```python
from build123d import *

# Parameters (mm, degrees)
SKETCH_R      = 4
EXTRUDE_DEPTH = 10


with BuildPart() as part:
    # Sketch → Extrude (new body)
    with BuildSketch(Plane.XY):
        with BuildLine():
            Line((18.316745, 55.716924), (18.316745, 0.716924))
            Line((18.316745, 0.716924), (23.316745, 0.716924))
            Line((23.316745, 0.716924), (23.316745, 14.716924))
            Line((23.316745, 14.716924), (33.741258, 14.716924))
            ThreePointArc((33.741258, 14.716924), (42.987024, 18.546645), (46.816745, 27.792411))
            Line((46.816745, 27.792411), (46.816745, 28.641436))
            ThreePointArc((46.816745, 28.641436), (42.987024, 37.887202), (33.741258, 41.716924))
            Line((33.741258, 41.716924), (23.316745, 41.716924))
            Line((23.316745, 41.716924), (23.316745, 55.716924))
            Line((23.316745, 55.716924), (18.316745, 55.716924))
        make_face()
        with Locations((33.316745, 28.216924)):
            Circle(SKETCH_R, mode=Mode.SUBTRACT)
    extrude(amount=EXTRUDE_DEPTH)


solid = part.part
```
Geometry: final body of the model. Coordinates: model frame, mm. A direction names the side the tool comes from. Round coordinates to 2 decimals unless told otherwise and drop trailing zeros. Order: outer loops, then holes, each group sorted by start corner. A loop starts at its lowest first (then second) coordinate and runs counter-clockwise, first axis right, second up. Notation, with made-up numbers: (-29.5, 36) -> (-3.5, 36) arc R23 ccw to (-3.5, 56) -> close; hole circle Ø5 at (-19, 9.25). An arc over 180 degrees is marked (long way). Use CSV: the item, a comma, the result in double quotes. Start each with the question number.
1) Section A-A (z = 3). Return the cut outline in (x, y).
2) Material intervals for line 1 along X through (y, z) = (39, 4); line 2 along X through (y, z) = (43, 2); line 3 along Y through (x, z) = (36, 1.5), sorted ascending. Write a range as from..to.
3) Draft query along X for faces 4 (the face through (29, 29, 0)), 5 (the face through (42.885, 18.446, 4.93)), 6 (the face through (18.317, 29, 5)), 7 (the face through (30.142, 25.783, 4.93)). Return one class per face: +X half, -X half, draft (parallel to the pull), parting line (faces both ways), or undercut.
4) First-contact query: pin 1 Ø5 at (x, z) = (27.5, 4.5) entering from -Y; pin 2 Ø1 at (y, z) = (23, 7.5) entering from +X; pin 3 Ø3 at (y, z) = (5.5, 5.5) entering from +X. Flat tips, straight axial feed; report the tip coordinate or a pass-through.
5) Set-up query: faces 1 (the face through (21, 0.717, 5)), 2 (the face through (23.317, 49, 5)), 3 (the face through (23.317, 8, 5)). Return all of +Z, -Z, +X, -X, +Y, -Y with unobstructed straight access to the full face (end or side cutting, diameter ignored); none if empty.
6) Section D-D (x = 44.75). Return the cut outline in (y, z), and give its area (3 significant figures).
7) Section B-B (x = 31). Return the cut outline in (y, z), and give its area (3 significant figures).
8) Section C-C (y = 10). Return the cut outline in (x, z), and give its area (3 significant figures).
Returned:
1,outline,"(18.32, 0.72) -> (23.32, 0.72) -> (23.32, 14.72) -> (33.74, 14.72) arc R13.08 ccw to (46.82, 27.79) -> (46.82, 28.64) arc R13.08 ccw to (33.74, 41.72) -> (23.32, 41.72) -> (23.32, 55.72) -> (18.32, 55.72) -> close; hole circle Ø8 at (33.32, 28.22)"
2,line 1,"x = 18.32..41.72"
2,line 2,"x = 18.32..23.32"
2,line 3,"y = 14.91..25.25, 31.18..41.52"
3,face 4,"draft"
3,face 5,"+X half"
3,face 6,"-X half"
3,face 7,"undercut"
4,pin 1,"stops at y = 14.72"
4,pin 2,"stops at x = 46.09"
4,pin 3,"stops at x = 23.32"
5,face 1,"+Z, -Z, +X, -X, -Y"
5,face 2,"+Z, -Z, +X, +Y"
5,face 3,"+Z, -Z, +X, -Y"
6,outline,"(20.74, 0) -> (35.7, 0) -> (35.7, 10) -> (20.74, 10) -> close"
6,area,"150 mm²"
7,outline,"(14.72, 0) -> (24.96, 0) -> (24.96, 10) -> (14.72, 10) -> close; (31.48, 0) -> (41.72, 0) -> (41.72, 10) -> (31.48, 10) -> close"
7,area,"205 mm²"
8,outline,"(18.32, 0) -> (23.32, 0) -> (23.32, 10) -> (18.32, 10) -> close"
8,area,"50.0 mm²"
